The listing builds one solid part. Answer for the finished solid, in the listing's coordinates (mm). A direction names the side the tool comes from. Give positions to 0.01 mm unless a question says otherwise; leave off trailing zeros. Loops run counter-clockwise (first coordinate to the right, second up) from the corner with the lowest first, then second, coordinate; pieces in that order, holes last.
Item 1: The mould has two halves that part along Y. Classify faces 3 (the face through (11.52, 18.07, 1.57)), 4 (the face through (2, 22, 0)), 5 (the face through (-4.68, -21.07, 9.37)): pulls with the +Y half, pulls with the -Y half, needs draft (parallel to the pull), parting line crosses it, or undercut.
Item 2: Section D-D, the plane z = 7.5 is taken. Give the vertices of the cut face in (x, y).
Item 3: Each of these flat-tipped pins is pushed along its axis until it touches: pin 1 Ø4 at (x, y) = (-6, -1.5) entering from -Z; pin 2 Ø1.5 at (x, z) = (-14.5, 6.5) entering from -Y; pin 3 Ø2 at (y, z) = (-6, 3.5) entering from -X. Where does it stop, or does it pass through?
Item 4: Consider line 1 along Y through (x, z) = (0, 1.75); line 2 along Y through (x, z) = (0, 5.55) (3 decimals); line 3 along X through (y, z) = (-0.5, 6). Determine where each line is inside the solid, lowest interval first.
Item 5: Section A-A, the plane y = 0 is taken. Give the vertices of the cut face in (x, z) (3 decimals).
Item 6: A tool of negligible diameter and unlimited length cuts with its end or side. For faces 1 (the face through (4, -9, 3.175)), 2 (the face through (0, 0, 9.525)), from which of +Z, -Z, +X, -X, +Y, -Y can it reach the whole face along a straight path? Write none if from no direction.
from build123d import *

# Parameters (mm, degrees)
F0_R     = 24.60625
F1_DEPTH = 9.525
F2_R     = 21.43125
F3_DEPTH = 3.175
F4_R     = 9.525
F5_DEPTH = 3.175
F6_SIZE  = 3.175


with BuildPart() as f1:
    # F0 (on Top) → F1 (new body)
    with BuildSketch(Plane.XY):
        Circle(F0_R)
    extrude(amount=F1_DEPTH)

    # F2 (on face) → F3 (cut)
    with BuildSketch(Plane.XY):
        Circle(F2_R)
    extrude(amount=F3_DEPTH, mode=Mode.SUBTRACT)

    # F4 (on face) → F5 (cut)
    with BuildSketch(Plane(origin=(0, 0, 3.175), x_dir=(1, 0, 0), z_dir=(0, 0, -1))):
        Circle(F4_R)
    extrude(amount=-F5_DEPTH, mode=Mode.SUBTRACT)

    # F6
    f6_edges = [f1.edges().sort_by_distance(p)[0] for p in [
        (-24.60625, 0, 9.525),
    ]]
    chamfer(f6_edges, length=F6_SIZE)


solid = f1.part
Worked answers:
1. face 3: undercut
1. face 4: needs draft
1. face 5: parting line crosses it
2. outline: circle Ø46.91 at (0, 0)
3. pin 1: stops at z = 6.35
3. pin 2: stops at y = -20.4
3. pin 3: stops at x = -24.09
4. line 1: y = -24.61 to -21.43, 21.43 to 24.61
4. line 2: y = -24.606 to -9.525, 9.525 to 24.606
4. line 3: x = -24.6 to -9.51, 9.51 to 24.6
5. outline: (-24.606, 0) - (-21.431, 0) - (-21.431, 3.175) - (-9.525, 3.175) - (-9.525, 6.35) - (9.525, 6.35) - (9.525, 3.175) - (21.431, 3.175) - (21.431, 0) - (24.606, 0) - (24.606, 6.35) - (21.431, 9.525) - (-21.431, 9.525) - (-24.606, 6.35) - close
6. face 1: -Z
6. face 2: +Z, +X, -X, +Y, -Y
